```python
from build123d import *

# Parameters (mm, degrees)
BOSS_EXTRUDE1_DEPTH   = 30
F_3_0MM_DOWEL_HOLE1_D = 3.2
SKETCH6_R             = 2.5
CUT_EXTRUDE1_DEPTH    = 8


with BuildPart() as part:
    # Sketch1 → Boss-Extrude1 (new body)
    with BuildSketch(Plane(origin=(0, 0, 0), x_dir=(1, 0, 0), z_dir=(0, 1, 0))):
        Polygon((-6, -1.25), (-4.25, -1.25), (-4.25, -2.25), (-6, -2.25), (-6, -4), (-22.7, -4), (-22.7, 7), (22.7, 7), (22.7, -4), (6, -4), (6, -2.25), (4.25, -2.25), (4.25, -1.25), (6, -1.25), (6, 4), (-6, 4), align=None)
    extrude(amount=BOSS_EXTRUDE1_DEPTH)

    # Ø3.0mm Dowel Hole1 (through all)
    with Locations(Plane.XY.offset(4)):
        with Locations((-10, 25), (10, 25), (10, 5), (-10, 5)):
            Hole(F_3_0MM_DOWEL_HOLE1_D / 2)

    # Sketch6 → Cut-Extrude1 (cut)
    with BuildSketch(Plane.XY.offset(4)):
        with Locations((9.5, 15)):
            Circle(SKETCH6_R)
        with Locations((-9.5, 15)):
            Circle(SKETCH6_R)
    extrude(amount=-CUT_EXTRUDE1_DEPTH, mode=Mode.SUBTRACT)


solid = part.part
```
Build history of the part. All positions in model axes, mm. A direction names the side the tool comes from. Give positions to 0.01 mm unless a question says otherwise; leave off trailing zeros. Loops run counter-clockwise (first coordinate to the right, second up) from the corner with the lowest first, then second, coordinate; pieces in that order, holes last.
1) Band-saw the part on A-A on z = -2.75. List the corners of the cut face in (x, y).
Values follow:
outline: (-22.7, 0) - (-6, 0) - (-6, 30) - (-22.7, 30) - close; (6, 0) - (22.7, 0) - (22.7, 30) - (6, 30) - close; hole circle Ø5 at (-9.5, 15); hole circle Ø3.2 at (-10, 5); hole circle Ø3.2 at (-10, 25); hole circle Ø5 at (9.5, 15); hole circle Ø3.2 at (10, 5); hole circle Ø3.2 at (10, 25)
2) Probe line 1 along X through (y, z) = (20.25, -3.5); line 2 along Z through (x, y) = (-4.5, 8); line 3 along Y through (x, z) = (9.5, -2). List the from-to ranges inside material, lowest first.
Values follow:
line 1: x = -22.7 to -6, 6 to 22.7
line 2: z = -7 to -4, 1.25 to 2.25
line 3: y = 0 to 3.48, 6.52 to 12.5, 17.5 to 23.48, 26.52 to 30
3) Drop flat-ended pins along their axis: P1, Ø0.5, axis at x = 5.5, y = 11.5, coming from the +Z side; P2, Ø6, axis at x = 7, z = 0.5, coming from the -Y side; P3, Ø1.9, axis at x = -10, y = 25, coming from the -Z side. Give the stop position or say it passes through.
Values follow:
P1: stops at z = 2.25
P2: stops at y = 0
P3: passes through
4) Band-saw the part on C-C on y = 25. List the corners of the cut face in (x, z).
Values follow:
outline: (-22.7, -7) - (-11.6, -7) - (-11.6, 4) - (-22.7, 4) - close; (-8.4, -7) - (8.4, -7) - (8.4, 4) - (6, 4) - (6, 2.25) - (4.25, 2.25) - (4.25, 1.25) - (6, 1.25) - (6, -4) - (-6, -4) - (-6, 1.25) - (-4.25, 1.25) - (-4.25, 2.25) - (-6, 2.25) - (-6, 4) - (-8.4, 4) - close; (11.6, -7) - (22.7, -7) - (22.7, 4) - (11.6, 4) - close
5) Two-plate mould, pull along X, no slides. Class faces 5 (the face through (-22.7, 15, -1)), 6 (the face through (-14, 15, 4)), 7 (the face through (-6, 15, 3)): released by +X, released by -X, zero draft, split by the parting line, or undercut.
Values follow:
face 5: released by -X
face 6: zero draft
face 7: undercut
6) 3-axis set-ups, long thin cutter, end or side, ignore diameter. For faces 1 (the face through (-5, 15, 2.25)), 2 (the face through (14, 15, 4)), 3 (the face through (8.96, 12.56, 0.06)), 4 (the face through (0, 15, -4)): which of +Z, -Z, +X, -X, +Y, -Y reach the whole face in a straight line?
Values follow:
face 1: +Z, +Y, -Y
face 2: +Z, +X, -X, +Y, -Y
face 3: +Z
face 4: +Y, -Y
7) Band-saw the part on B-B on x = 5.5. List the corners of the cut face in (y, z).
Values follow:
outline: (0, -7) - (30, -7) - (30, -4) - (0, -4) - close; (0, 1.25) - (30, 1.25) - (30, 2.25) - (0, 2.25) - close
8) Band-saw the part on D-D on z = -6. List the corners of the cut face in (x, y), then the cut area to 3 significant figures.
Values follow:
outline: (-22.7, 0) - (22.7, 0) - (22.7, 30) - (-22.7, 30) - close; hole circle Ø3.2 at (-10, 5); hole circle Ø3.2 at (-10, 25); hole circle Ø3.2 at (10, 5); hole circle Ø3.2 at (10, 25)
area: 1,330 mm2
